```python
from build123d import *

# Parameters (mm, degrees)
F0_R     = 2.675
F1_DEPTH = 7.5
F0_R_2   = 2.3375
F2_W     = 15
F2_H     = 7
F2_R     = 2.3375
F2_H_2   = 12.555
F2_H_3   = 6.5
F3_DEPTH = 3
F4_R     = 5


# Not quite as in the source:
# - a feature names something its author has since deleted; it is built from what else it names


with BuildPart() as f1:
    # F0 (on Top) → F1 (new body)
    with BuildSketch(Plane.XY):
        Circle(F0_R)
    extrude(amount=F1_DEPTH)



with BuildPart() as f1b:
    # F0 (on Top) → F1, piece 2 (new body)
    with BuildSketch(Plane.XY):
        with Locations((0, 19.305)):
            Circle(F0_R_2)
    extrude(amount=F1_DEPTH)


with BuildPart() as f1_1:
    add(f1.part)

    add(f1b.part)  # F3 merges F1b
    # F2 (on face) → F3 (join)
    with BuildSketch(Plane.XY.offset(7.5)):
        with Locations((0, 19.305)):
            Rectangle(F2_W, F2_H)
        with Locations((0, 19.305)):
            Circle(F2_R, mode=Mode.SUBTRACT)
        with Locations((0, 19.305)):
            Circle(F2_R)
        with Locations((0, 9.5275)):
            Rectangle(F2_W, F2_H_2)
        Rectangle(F2_W, F2_H_3)
    extrude(amount=F3_DEPTH)

    # F4
    f4_edges = [f1_1.edges().sort_by_distance(p)[0] for p in [
        (-7.5, -3.25, 9),
        (7.5, -3.25, 9),
        (7.5, 22.805, 9),
        (-7.5, 22.805, 9),
    ]]
    fillet(f4_edges, radius=F4_R)


solid = f1_1.part
```
Could you check a few things on this model? Use its own coordinates, in mm. A direction names the side the tool comes from. Give positions to 0.01 mm unless a question says otherwise; leave off trailing zeros. Loops run counter-clockwise (first coordinate to the right, second up) from the corner with the lowest first, then second, coordinate; pieces in that order, holes last. Notation, with made-up numbers: (71, 26.5) -> (96, 26.5) arc R23 ccw to (96, 48.5) -> close; hole circle Ø11 at (28, 86). An arc over 180 degrees is marked (long way). Put each result on its own line as item: value.
(1) Imagine slicing it at B-B on z = 8. Write out the boundary of the cut face in (x, y) (3 decimals), plus the area to 3 significant figures.
Computed:
outline: (-7.5, 1.75) arc R5 ccw to (-2.5, -3.25) -> (2.5, -3.25) arc R5 ccw to (7.5, 1.75) -> (7.5, 17.805) arc R5 ccw to (2.5, 22.805) -> (-2.5, 22.805) arc R5 ccw to (-7.5, 17.805) -> close
area: 369 mm^2
(2) For faces 1 (the face through (-0.58, -2.61, 3.7)), 2 (the face through (7.5, 10, 9)), which set-ups out of +Z, -Z, +X, -X, +Y, -Y let a thin tool reach every point of the face, with its end or its side?
Computed:
face 1: -Z
face 2: +Z, -Z, +X, +Y, -Y
(3) I'm going to push flat-ended pins straight in: pin 1 Ø3 at (x, y) = (-5.5, 10) entering from -Z; pin 2 Ø3 at (x, z) = (3.5, 3.5) entering from -Y; pin 3 Ø3 at (y, z) = (4.5, 1) entering from -X. Where does each tip first touch, or does it pass through?
Computed:
pin 1: z = 7.5
pin 2: y = -1.78
pin 3: through
(4) Thinking about a two-plate mould opening in Y: for faces 3 (the face through (-7.5, 10, 9)), 4 (the face through (0, 10, 7.5)), 5 (the face through (-6.07, -1.75, 9.02)), which applies, pulls with the +Y half, pulls with the -Y half, needs draft (parallel to the pull), parting line crosses it, or undercut?
Computed:
face 3: needs draft
face 4: undercut
face 5: pulls with the -Y half
(5) Imagine slicing it at C-C on y = 1. Write out the boundary of the cut face in (x, z).
Computed:
outline: (-7.44, 7.5) -> (-2.48, 7.5) -> (-2.48, 0) -> (2.48, 0) -> (2.48, 7.5) -> (7.44, 7.5) -> (7.44, 10.5) -> (-7.44, 10.5) -> close
(6) Please list where these lines run through material, in increasing order: probe 1 along Z at (x, y) = (6.75, 0); probe 2 along Y at (x, z) = (-5.5, 9.75) (3 decimals); probe 3 along X at (y, z) = (19.75, 8.5). Write a range as [from, to].
Computed:
probe 1: [7.5, 10.5]
probe 2: [-2.25, 21.805]
probe 3: [-7.11, 7.11]
